Can you work these out from the model? Positions are in its coordinate system, mm. Give positions to 0.01 mm unless a question says otherwise; leave off trailing zeros. Loops run counter-clockwise (first coordinate to the right, second up) from the corner with the lowest first, then second, coordinate; pieces in that order, holes last. Notation, with made-up numbers: (-2.5, 82.5) - (32.5, 82.5) arc R17 ccw to (32.5, 102.5) - close; hole circle Ø5 at (33, -37). An arc over 180 degrees is marked (long way). Write item = value, one per line.
from build123d import *

# Parameters (mm, degrees)
F0_W     = 50.8
F0_H     = 6.35
F1_DEPTH = 165.1
F2_R     = 2.5019
F2_R_2   = 2.6162
F3_DEPTH = 6.351


with BuildPart() as f1:
    # F0 (on Front) → F1 (new body)
    with BuildSketch(Plane.XZ):
        Rectangle(F0_W, F0_H)
    extrude(amount=F1_DEPTH)

    # F2 (on face) → F3 (cut, through all)
    with BuildSketch(Plane.XY.offset(3.175)):
        with Locations((-20.0025, -94.5515)):
            Circle(F2_R)
        with Locations((20.0025, -94.5515)):
            Circle(F2_R)
        with Locations((20.0025, -70.5485)):
            Circle(F2_R)
        with Locations((-20.0025, -70.5485)):
            Circle(F2_R)
        with Locations((-19.05, -139.7)):
            Circle(F2_R_2)
        with Locations((19.05, -139.7)):
            Circle(F2_R_2)
        with Locations((-19.05, -25.4)):
            Circle(F2_R_2)
        with Locations((19.05, -25.4)):
            Circle(F2_R_2)
    extrude(amount=-F3_DEPTH, mode=Mode.SUBTRACT)


solid = f1.part
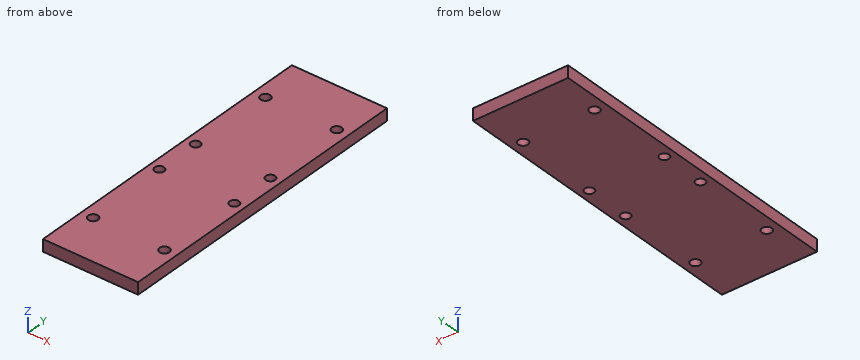
Q1. Imagine slicing it at B-B, the plane x = 19.05. Write out the boundary of the cut face in (y, z) (3 decimals), then the cut area to 3 significant figures.
Output:
outline = (-165.1, -3.175) - (-142.316, -3.175) - (-142.316, 3.175) - (-165.1, 3.175) - close; (-137.084, -3.175) - (-96.865, -3.175) - (-96.865, 3.175) - (-137.084, 3.175) - close; (-92.238, -3.175) - (-72.862, -3.175) - (-72.862, 3.175) - (-92.238, 3.175) - close; (-68.235, -3.175) - (-28.016, -3.175) - (-28.016, 3.175) - (-68.235, 3.175) - close; (-22.784, -3.175) - (0, -3.175) - (0, 3.175) - (-22.784, 3.175) - close
area = 923 mm2
Q2. Imagine slicing it at A-A, the plane y = -139.7. Write out the boundary of the cut face in (x, z) (3 decimals), then the cut area to 3 significant figures.
Output:
outline = (-25.4, -3.175) - (-21.666, -3.175) - (-21.666, 3.175) - (-25.4, 3.175) - close; (-16.434, -3.175) - (16.434, -3.175) - (16.434, 3.175) - (-16.434, 3.175) - close; (21.666, -3.175) - (25.4, -3.175) - (25.4, 3.175) - (21.666, 3.175) - close
area = 256 mm2
Q3. Imagine slicing it at C-C, the plane z = -2. Give the number of separate pieces and of enclosed holes in the cut face, then the cut area to 3 significant figures.
Output:
separate_pieces = 1
enclosed_holes = 8
area = 8,220 mm2
Q4. For pin 1 (8 mm diameter, centred on x = 20, y = -94.55, fed in from -Z) (3 decimals); pin 2 (4.5 mm diameter, centred on x = 20, y = -70.55, fed in from +Z), each with a flat end and sliding along its axis, tell me the tip position at first contact or that it passes through.
Output:
pin_1 = -3.175
pin_2 = through
Q5. I need wall thicknesses on L1, parallel to Y at x = 22, z = -0.75; L2, parallel to Y at x = -19.05, z = 2 (3 decimals); L3, parallel to Y at x = 20, z = 0.25. Which ranges of each line are inside material? Lowest first, please.
Output:
L1 = -165.1 to -96.06, -93.05 to -72.05, -69.04 to 0
L2 = -165.1 to -142.316, -137.084 to -96.865, -92.238 to -72.862, -68.235 to -28.016, -22.784 to 0
L3 = -165.1 to -142.14, -137.26 to -97.05, -92.05 to -73.05, -68.05 to -27.84, -22.96 to 0
